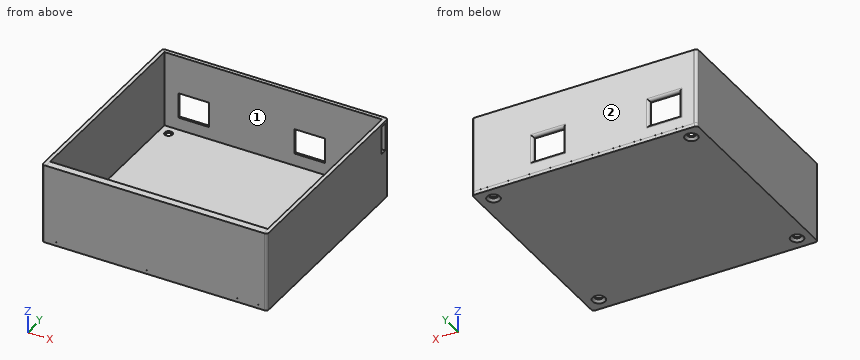
from build123d import *

# Parameters (mm, degrees)
BOX_W            = 20
BOX_H            = 2.5
BOX_DEPTH        = 11
SKETCH005_W      = 12
SKETCH005_H      = 10
EXTRUDE008_DEPTH = 1.5
SKETCH002_W      = 84.01
SKETCH002_H      = 30
EXTRUDE002_DEPTH = 1.5
FILLET001_R      = 1
FILLET003_R      = 1
SKETCH003_W      = 84.01
SKETCH003_H      = 30
EXTRUDE007_DEPTH = 1.5
FILLET005_R      = 1
SKETCH001_W      = 89
SKETCH001_H      = 84
SKETCH001_R      = 1.524
EXTRUDE001_DEPTH = 1.5
FILLET_R         = 1
FILLET002_R      = 1
FILLET004_R      = 1
FILLET006_R      = 1
EXTRUDE004_DEPTH = 3
FILLET011_R      = 1
CHAMFER_SIZE     = 1
CHAMFER001_SIZE  = 1
CHAMFER002_SIZE  = 1
CHAMFER003_SIZE  = 1
FILLET016_R      = 1
FILLET017_R      = 1


with BuildPart() as box:
    # Box → Box (new body)
    with BuildSketch(Plane(origin=(134, 92, 18), x_dir=(1, 0, 0), z_dir=(0, 0, 1))):
        with Locations((10, 1.25)):
            Rectangle(BOX_W, BOX_H)
    extrude(amount=BOX_DEPTH)


with BuildPart() as extrude008:
    # Sketch005 → Extrude008 (new body)
    with BuildSketch(Plane.XZ):
        Polygon((48.658601, 30.00186), (134.672964, 30.001823), (134.673007, -0.086485), (48.658601, -0.081194), align=None)
        with Locations((60.167907, 9.918134)):
            Rectangle(SKETCH005_W, SKETCH005_H, mode=Mode.SUBTRACT)
        with Locations((106.097198, 9.915282)):
            Rectangle(SKETCH005_W, SKETCH005_H, mode=Mode.SUBTRACT)
    extrude(amount=EXTRUDE008_DEPTH)


with BuildPart() as extrude008_1:
    # Extrude008 placement: moved
    add(extrude008.part.moved(Location((0.009309, 96.402171, 0.006059))))


with BuildPart() as fillet003:
    # Sketch002 → Extrude002 (new body)
    with BuildSketch(Plane.YZ):
        with Locations((54.387171, 15)):
            Rectangle(SKETCH002_W, SKETCH002_H)
    extrude(amount=EXTRUDE002_DEPTH)


with BuildPart() as fillet003_1:
    # Extrude002 placement: moved
    add(fillet003.part.moved(Location((47.167907, 0.01, 0))))

    # Fillet001
    fillet001_edges = [fillet003_1.edges().sort_by_distance(p)[0] for p in [
        (47.167907, 96.402171, 15),
    ]]
    fillet(fillet001_edges, radius=FILLET001_R)

    # Fillet003
    fillet003_edges = [fillet003_1.edges().sort_by_distance(p)[0] for p in [
        (47.167907, 12.392171, 15),
    ]]
    fillet(fillet003_edges, radius=FILLET003_R)


with BuildPart() as fillet005:
    # Sketch003 → Extrude007 (new body)
    with BuildSketch(Plane.YZ):
        with Locations((54.387171, 15)):
            Rectangle(SKETCH003_W, SKETCH003_H)
    extrude(amount=EXTRUDE007_DEPTH)


with BuildPart() as fillet005_1:
    # Extrude007 placement: moved
    add(fillet005.part.moved(Location((134.667907, 0.01, 0))))

    # Fillet005
    fillet005_edges = [fillet005_1.edges().sort_by_distance(p)[0] for p in [
        (136.167907, 12.392171, 15),
    ]]
    fillet(fillet005_edges, radius=FILLET005_R)


with BuildPart() as fillet006:
    # Sketch001 → Extrude001 (new body)
    with BuildSketch(Plane.XY):
        with Locations((91.667907, 54.392171)):
            Rectangle(SKETCH001_W, SKETCH001_H)
        with Locations((52.453907, 91.106708)):
            Circle(SKETCH001_R, mode=Mode.SUBTRACT)
        with Locations((130.657907, 91.102171)):
            Circle(SKETCH001_R, mode=Mode.SUBTRACT)
        with Locations((130.707907, 17.767171)):
            Circle(SKETCH001_R, mode=Mode.SUBTRACT)
        with Locations((52.453907, 17.678171)):
            Circle(SKETCH001_R, mode=Mode.SUBTRACT)
    extrude(amount=-EXTRUDE001_DEPTH)

    # Fillet
    fillet_edges = [fillet006.edges().sort_by_distance(p)[0] for p in [
        (47.167907, 96.392171, -0.75),
    ]]
    fillet(fillet_edges, radius=FILLET_R)

    # Fillet002
    fillet002_edges = [fillet006.edges().sort_by_distance(p)[0] for p in [
        (47.167907, 12.392171, -0.75),
    ]]
    fillet(fillet002_edges, radius=FILLET002_R)

    # Fillet004
    fillet004_edges = [fillet006.edges().sort_by_distance(p)[0] for p in [
        (136.167907, 12.392171, -0.75),
    ]]
    fillet(fillet004_edges, radius=FILLET004_R)

    # Fillet006
    fillet006_edges = [fillet006.edges().sort_by_distance(p)[0] for p in [
        (136.167907, 96.392171, -0.75),
    ]]
    fillet(fillet006_edges, radius=FILLET006_R)


with BuildPart() as fillet017:
    # Sketch004 (on Sketch) → Extrude004 (new body)
    with BuildSketch(Plane.XZ):
        Polygon((48.658598, 30.00186), (134.672964, 30.001823), (134.672964, -0.003143), (48.658598, -0.006059), align=None)
    extrude(amount=EXTRUDE004_DEPTH)


with BuildPart() as fillet017_1:
    # Extrude004 placement: moved
    add(fillet017.part.moved(Location((0.009309, 15.392171, 0.006059))))

    # Fusion: union Extrude008, Fillet003, Fillet005, Fillet006
    add(extrude008_1.part)
    add(fillet003_1.part)
    add(fillet005_1.part)
    add(fillet006.part)

    # Fillet011
    fillet011_edges = [fillet017_1.edges().sort_by_distance(p)[0] for p in [
        (136.167907, 96.402171, 15),
    ]]
    fillet(fillet011_edges, radius=FILLET011_R)

    # Chamfer
    chamfer_edges = [fillet017_1.edges().sort_by_distance(p)[0] for p in [
        (50.929907, 17.678171, -1.5),
    ]]
    chamfer(chamfer_edges, length=CHAMFER_SIZE)

    # Chamfer001
    chamfer001_edges = [fillet017_1.edges().sort_by_distance(p)[0] for p in [
        (129.183907, 17.767171, -1.5),
    ]]
    chamfer(chamfer001_edges, length=CHAMFER001_SIZE)

    # Chamfer002
    chamfer002_edges = [fillet017_1.edges().sort_by_distance(p)[0] for p in [
        (129.133907, 91.102171, -1.5),
    ]]
    chamfer(chamfer002_edges, length=CHAMFER002_SIZE)

    # Chamfer003
    chamfer003_edges = [fillet017_1.edges().sort_by_distance(p)[0] for p in [
        (50.929907, 91.106708, -1.5),
    ]]
    chamfer(chamfer003_edges, length=CHAMFER003_SIZE)

    # Cut: cut Box
    add(box.part, mode=Mode.SUBTRACT)

    # Fillet016
    fillet016_edges = [fillet017_1.edges().sort_by_distance(p)[0] for p in [
        (106.106507, 96.402171, 14.921341),
        (100.106507, 96.402171, 9.921341),
        (106.106507, 96.402171, 4.921341),
        (112.106507, 96.402171, 9.921341),
    ]]
    fillet(fillet016_edges, radius=FILLET016_R)

    # Fillet017
    fillet017_edges = [fillet017_1.edges().sort_by_distance(p)[0] for p in [
        (60.177215, 96.402171, 14.924193),
        (54.177215, 96.402171, 9.924193),
        (60.177215, 96.402171, 4.924193),
        (66.177215, 96.402171, 9.924193),
    ]]
    fillet(fillet017_edges, radius=FILLET017_R)


solid = fillet017_1.part
The model under review builds one solid part; all positions refer to its coordinate system, in mm. Face numbers are marked on the shaded views. A direction names the side the tool comes from. Coordinates: 2 decimals unless noted, no trailing zeros. Loops run counter-clockwise (first coordinate to the right, second up) from the corner with the lowest first, then second, coordinate; pieces in that order, holes last. Notation, with made-up numbers: (41.5, 44.25) -> (62.5, 44.25) arc R27 ccw to (62.5, 75.25) -> close; hole circle Ø10 at (-12.75, -9.75). An arc over 180 degrees is marked (long way). Use a Markdown table: item, result. Add a question column.
1. Add section D-D on y = 40.5. Write out the cut boundary in (x, z), plus the area to 4 significant figures.
2. To check wall thickness, follow line 1 (X direction, y = 17.5, z = 14); line 2 (Y direction, x = 57.5, z = 21.5); line 3 (Z direction, x = 107, y = 67). State the ranges of each line that lie inside material, in increasing order.
3. Machinability: for the marked faces 1 and 2, which of the approach directions +Z, -Z, +X, -X, +Y, -Y give a long, thin tool a straight path to every point of the face, cutting with its end or side? Answer none if there is none.
4. Clearance check with flat-ended pins moving along their axes: pin 1 Ø3 at (x, y) = (94, 88) entering from +Z; pin 2 Ø4 at (x, y) = (130.66, 91.1) entering from -Z. State where each tip first meets the part, or that it passes through.
Returned:
| question | item | result |
|---|---|---|
| 1 | outline | (47.17, -1.5) -> (136.17, -1.5) -> (136.17, 30) -> (134.67, 30) -> (134.67, 0) -> (48.67, 0) -> (48.67, 30) -> (47.17, 30) -> close |
| 1 | area | 223.5 mm² |
| 2 | line 1 | x = 47.17 to 48.67, 134.67 to 136.17 |
| 2 | line 2 | y = 12.39 to 15.39, 94.9 to 96.4 |
| 2 | line 3 | z = -1.5 to 0 |
| 3 | face 1 | +Z |
| 3 | face 2 | +Z, -Z, +X, -X, +Y |
| 4 | pin 1 | stops at z = 0 |
| 4 | pin 2 | stops at z = -0.98 |
